Input: part model. Units: mm. Frame: model coordinates. A direction names the side the tool comes from. Coordinates: 2 decimals unless noted, no trailing zeros. Loops run counter-clockwise (first coordinate to the right, second up) from the corner with the lowest first, then second, coordinate; pieces in that order, holes last. Notation, with made-up numbers: M 27.25,-30.75 L 56.25,-30.75 A18 cw 56.25,-16.75 Z; hole C 83.5,61.5 d2. An arc over 180 degrees is marked long. Use a Markdown table: item, result. Add a question column.
1. Section A-A on y = 79.5. Output: boundary loops of the cut face in (x, z), then the cut area to 3 significant figures.
2. Set-up query: faces 5 (the flat face through (89, 74, 50.8)), 6 (the flat face through (95, 88.9, 25)). Return all of +Z, -Z, +X, -X, +Y, -Y with unobstructed straight access to the full face (end or side cutting, diameter ignored); none if empty.
3. Line query: L1, parallel to Z at x = 70, y = 38.1; L2, parallel to X at y = 40, z = 4 (3 decimals); L3, parallel to X at y = 78.5, z = 36. Output: solid intervals per line, ascending. Write a range as [from, to].
4. Section D-D on y = 40.5. Output: boundary loops of the cut face in (x, z).
5. Pin query (flat end, axial travel): pin 1 (6 mm diameter, centred on x = 35, y = 69, fed in from -Z); pin 2 (4 mm diameter, centred on x = 34.5, z = 20.5, fed in from +Y); pin 3 (6.5 mm diameter, centred on x = 87, z = 56, fed in from +Y); pin 4 (20.5 mm diameter, centred on x = 19, y = 82.5, fed in from +Z). Return the tip coordinate at first contact, or that it passes through.
6. Draft query along X for faces 1 (the flat face through (0, 54, 38)), 2 (the flat face through (52, 35, 0)), 3 (the flat face through (69.58, 63.14, 31.31)), 4 (the flat face through (31.48, 63.86, 31.31)). Return one class per face: +X half, -X half, draft (parallel to the pull), parting line (faces both ways), or undercut.
7. Section B-B on z = 25.4. Output: boundary loops of the cut face in (x, y), then the cut area to 3 significant figures.
8. Section C-C on x = 92.5. Output: boundary loops of the cut face in (y, z).
```python
from build123d import *

# Parameters (mm, degrees)
BOSS_EXTRUDE1_DEPTH = 63.5
SKETCH2_R           = 19.05
CUT_EXTRUDE1_DEPTH  = 102.6
CUT_EXTRUDE2_DEPTH  = 12.7


with BuildPart() as part:
    # Sketch1 → Boss-Extrude1 (new body)
    with BuildSketch(Plane.XY):
        Polygon((0, 0), (0, 88.9), (12.7, 88.9), (50.8, 38.1), (88.9, 88.9), (101.6, 88.9), (101.6, 0), align=None)
    extrude(amount=BOSS_EXTRUDE1_DEPTH)

    # Sketch2 → Cut-Extrude1 (cut, through all)
    with BuildSketch(Plane(origin=(0, 0, 0), x_dir=(0, 0, -1), z_dir=(1, 0, 0))):
        with Locations((-25.4, 38.1)):
            Circle(SKETCH2_R)
    extrude(amount=CUT_EXTRUDE1_DEPTH, mode=Mode.SUBTRACT)

    # Sketch3 → Cut-Extrude2 (cut)
    with BuildSketch(Plane.XY.offset(63.5)):
        Polygon((0, 63.5), (31.75, 63.5), (12.7, 88.9), (0, 88.9), align=None)
        Polygon((69.85, 63.5), (101.6, 63.5), (101.6, 88.9), (88.9, 88.9), align=None)
    extrude(amount=-CUT_EXTRUDE2_DEPTH, mode=Mode.SUBTRACT)


solid = part.part
```
Answers below:
| question | item | result |
|---|---|---|
| 1 | outline | M 0,0 L 19.75,0 L 19.75,50.8 L 0,50.8 Z; M 81.85,0 L 101.6,0 L 101.6,50.8 L 81.85,50.8 Z |
| 1 | area | 2,010 mm² |
| 2 | face 5 | +Z, +X, -X, +Y |
| 2 | face 6 | +Z, -Z, +X, -X, +Y |
| 3 | L1 | z = [0, 6.35], [44.45, 63.5] |
| 3 | L2 | x = [0, 49.375], [52.225, 101.6] |
| 3 | L3 | x = [0, 20.5], [81.1, 101.6] |
| 4 | outline | M 0,0 L 49,0 L 49,6.5 L 0,6.5 Z; M 0,44.3 L 49,44.3 L 49,63.5 L 0,63.5 Z; M 52.6,0 L 101.6,0 L 101.6,6.5 L 52.6,6.5 Z; M 52.6,44.3 L 101.6,44.3 L 101.6,63.5 L 52.6,63.5 Z |
| 5 | pin 1 | passes through |
| 5 | pin 2 | stops at y = 62.5 |
| 5 | pin 3 | stops at y = 63.5 |
| 5 | pin 4 | stops at z = 50.8 |
| 6 | face 1 | -X half |
| 6 | face 2 | draft |
| 6 | face 3 | undercut |
| 6 | face 4 | undercut |
| 7 | outline | M 0,0 L 101.6,0 L 101.6,19.05 L 0,19.05 Z; M 0,57.15 L 36.51,57.15 L 12.7,88.9 L 0,88.9 Z; M 65.09,57.15 L 101.6,57.15 L 101.6,88.9 L 88.9,88.9 Z |
| 7 | area | 3,500 mm² |
| 8 | outline | M 0,0 L 88.9,0 L 88.9,50.8 L 63.5,50.8 L 63.5,63.5 L 0,63.5 Z; hole C 38.1,25.4 d38.1 |
